Can you work these out from the model? Positions are in its coordinate system, mm. A direction names the side the tool comes from. Round coordinates to 2 decimals unless told otherwise and drop trailing zeros. Order: outer loops, then holes, each group sorted by start corner. A loop starts at its lowest first (then second) coordinate and runs counter-clockwise, first axis right, second up.
Q1. Will these pins go through, and if not, where does the flat tip stop? P1, Ø5, axis at x = -2.5, y = -5.5, coming from the +Z side; P2, Ø1, axis at x = -2.5, y = -1.5, coming from the +Z side; P3, Ø2, axis at x = 3.5, y = -4, coming from the +Z side; P4, Ø0.8, axis at x = 0, z = -4.5, coming from the -Y side.
Q2. If I drill on line 1 (Y direction, x = -4, z = -3.75); line 2 (Y direction, x = -0.5, z = -1.5); line 3 (Z direction, x = -1.5, y = 6.25), over which ranges is the centre line in solid material (lowest first)?
Q3. If we section it at D-D (y = 5.75): Please give me the cut outline in (x, z).
Q4. If we section it at A-A (z = 0): Please give me the cut outline in (x, y), plus the area to 4 significant figures.
Q5. If we section it at C-C (y = -8.5): Please give me the cut outline in (x, z), plus the area to 3 significant figures.
Q6. If we section it at B-B (x = 0): Please give me the cut outline in (y, z).
Q7. We'd pull the mould along Z, two halves only. Please class faces 1 (the face through (0, -5, -4)), 2 (the face through (-0.434, -7.746, -1.952)), 3 (the face through (2.2, -7.5, 0.1)): pulls with the +Z half, pulls with the -Z half, needs draft (parallel to the pull), parting line crosses it, or undercut.
Q8. For faces 4 (the face through (0, 8, -2)), 5 (the face through (0, 0, -6)), 6 (the face through (0, -2.5, -4.5)), which set-ups out of +Z, -Z, +X, -X, +Y, -Y let a thin tool reach every point of the face, with its end or its side?
from build123d import *

# Parameters (mm, degrees)
F1_DEPTH = 7.5
F2_R     = 0.5
F3_DEPTH = 4
F4_R     = 2
F5_DEPTH = 0.5
F6_R     = 2
F7_DEPTH = 1
F8_R     = 0.5
F9_DEPTH = 5


with BuildPart() as f1:
    # F0 (on Front) → F1 (new body, symmetric)
    with BuildSketch(Plane.XZ):
        with BuildLine():
            Line((-5, 3.316625), (-5, -3.316625))
            ThreePointArc((-5, -3.316625), (0, -6), (5, -3.316625))
            Line((5, -3.316625), (5, 3.316625))
            ThreePointArc((5, 3.316625), (0, 6), (-5, 3.316625))
        make_face()
    extrude(amount=F1_DEPTH, both=True)

    # F2 (on face) → F3 (join)
    with BuildSketch(Plane.XZ.offset(7.5)):
        Circle(F2_R)
    extrude(amount=F3_DEPTH)

    # F4 (on face) → F5 (join)
    with BuildSketch(Plane.XZ.offset(7.5)):
        Circle(F4_R)
    extrude(amount=F5_DEPTH)

    # F6 (on face) → F7 (join)
    with BuildSketch(Plane(origin=(0, 7.5, 0), x_dir=(-1, 0, 0), z_dir=(0, 1, 0))):
        Circle(F6_R)
    extrude(amount=F7_DEPTH)

    # F8 (on face) → F9 (cut)
    with BuildSketch(Plane.XZ.offset(7.5)):
        with Locations((0, 4.5)):
            Circle(F8_R)
        with Locations((0, -4.5)):
            Circle(F8_R)
    extrude(amount=-F9_DEPTH, mode=Mode.SUBTRACT)


solid = f1.part
Solution:
1. P1: stops at z = 6
1. P2: stops at z = 5.66
1. P3: stops at z = 5.45
1. P4: stops at y = -2.5
2. line 1: y = -7.5 to 7.5
2. line 2: y = -8 to 8.5
2. line 3: z = -5.81 to 5.81
3. outline: (-5, -3.32) arc R6 ccw to (5, -3.32) - (5, 3.32) arc R6 ccw to (-5, 3.32) - close
4. outline: (-5, -7.5) - (-2, -7.5) - (-2, -8) - (-0.5, -8) - (-0.5, -11.5) - (0.5, -11.5) - (0.5, -8) - (2, -8) - (2, -7.5) - (5, -7.5) - (5, 7.5) - (2, 7.5) - (2, 8.5) - (-2, 8.5) - (-2, 7.5) - (-5, 7.5) - close
4. area: 159.5 mm2
5. outline: circle Ø1 at (0, 0)
5. area: 0.785 mm2
6. outline: (-11.5, -0.5) - (-8, -0.5) - (-8, -2) - (-7.5, -2) - (-7.5, -4) - (-2.5, -4) - (-2.5, -5) - (-7.5, -5) - (-7.5, -6) - (7.5, -6) - (7.5, -2) - (8.5, -2) - (8.5, 2) - (7.5, 2) - (7.5, 6) - (-7.5, 6) - (-7.5, 5) - (-2.5, 5) - (-2.5, 4) - (-7.5, 4) - (-7.5, 2) - (-8, 2) - (-8, 0.5) - (-11.5, 0.5) - close
7. face 1: undercut
7. face 2: parting line crosses it
7. face 3: needs draft
8. face 4: +Y
8. face 5: -Z, +Y, -Y
8. face 6: -Y
